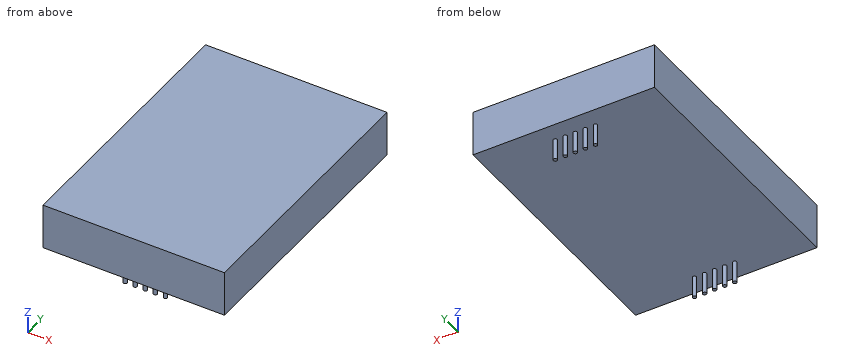
```python
from build123d import *

# Parameters (mm, degrees)
SKETCH_W            = 47.8
SKETCH_H            = 69.7
PAD_DEPTH           = 12
SKETCH001_R         = 0.5
PAD001_DEPTH        = 5.6
LINEARPATTERN_COUNT = 5
LINEARPATTERN_PITCH = 2.65


with BuildPart() as part:
    # Sketch → Pad (new body)
    with BuildSketch(Plane.XY):
        with Locations((-7.772954, 16.789133)):
            Rectangle(SKETCH_W, SKETCH_H)
    extrude(amount=PAD_DEPTH)

    # Sketch001 → Pad001 (new body)
    with BuildSketch(Plane(origin=(0, 0, 0), x_dir=(1, 0, 0), z_dir=(0, 0, -1))):
        with Locations((-13.072954, 13.060867)):
            Circle(SKETCH001_R)
        with Locations((-13.072954, -46.639133)):
            Circle(SKETCH001_R)
    pad001 = extrude(amount=PAD001_DEPTH)

    # LinearPattern: Pad001 ×5
    with Locations(*[(i * LINEARPATTERN_PITCH, 0, 0) for i in range(1, LINEARPATTERN_COUNT)]):
        add(pad001)


solid = part.part
```
Can you work these out from the model? Positions are in its coordinate system, mm. Coordinates: 2 decimals unless noted, no trailing zeros. Order: outer loops, then holes, each group sorted by start corner. A loop starts at its lowest first (then second) coordinate and runs counter-clockwise, first axis right, second up.
1. I need wall thicknesses on line 1 (Z direction, x = -28, y = 0.5). Which ranges of the line are inside material? Lowest first, please.
2. If we section it at B-B (y = -2.5): Please give me the cut outline in (x, z).
3. If we section it at A-A (z = -2.75): Give the number of separate pieces and of enclosed holes in the cut face, then the cut area to 3 significant figures.
4. If we section it at C-C (x = -24): Please give me the cut outline in (y, z).
5. I'm going to push a flat-ended pin straight in: pin 1 (6 mm diameter, centred on x = 5.5, y = 5.5, fed in from -Z). Where does the tip first touch, or does it pass through?
Entries:
1. line 1: z = 0 to 12
2. outline: (-31.67, 0) - (16.13, 0) - (16.13, 12) - (-31.67, 12) - close
3. separate pieces: 10
3. enclosed holes: 0
3. area: 7.85 mm2
4. outline: (-18.06, 0) - (51.64, 0) - (51.64, 12) - (-18.06, 12) - close
5. pin 1: stops at z = 0
